For this review, take the finished solid that the model builds, in its own axes (mm). Give positions to 0.01 mm unless a question says otherwise; leave off trailing zeros. Order: outer loops, then holes, each group sorted by start corner. A loop starts at its lowest first (then second) coordinate and runs counter-clockwise, first axis right, second up. Notation, with made-up numbers: (38.25, 12.25) -> (80.25, 12.25) arc R26 cw to (80.25, 28.25) -> close; hole circle Ø10 at (-6.75, -34). An arc over 180 degrees is marked (long way). One line per item, written item: value. Start each with the question number.
from build123d import *

# Parameters (mm, degrees)
F0_R     = 38.1
F1_DEPTH = 101.6
F2_T     = -2.54


# Not quite as in the source:
# - a fillet or chamfer that OpenCascade refuses, or shapes differently, is made with other operations: its cross-section is extruded or revolved along the edge and cut away or added


with BuildPart() as f1:
    # F0 (on Top) → F1 (new body)
    with BuildSketch(Plane.XY):
        Circle(F0_R)
    extrude(amount=F1_DEPTH)

    # F2
    f2_openings = [f1.faces().sort_by_distance(p)[0] for p in [
        (0, 0, 101.6),
    ]]
    offset(amount=F2_T, openings=f2_openings)

    # F3: fillet of radius 5.08 on 1 edges, made by hand

    # F3_s1 → F3_t2 (revolve, cut)
    with BuildSketch(Plane.XZ):
        with BuildLine():
            ThreePointArc((38.1, 97.2005909488), (37.4194090512, 99.7405909488), (35.56, 101.6))
            Line((35.56, 101.6), (38.1, 101.6))
            Line((38.1, 101.6), (38.1, 97.2005909488))
        make_face()
    revolve(axis=Axis((0, 0, 101.6), (0, 0, 1)), mode=Mode.SUBTRACT)


solid = f1.part
Q1. Take a section at C-C (z = 15). State the section outline as (x, y) points.
Q2. Mouldability with a two-part tool opening along Y and no side actions: class faces 1 (the flat face through (-1, 1, 0)), 2 (the cylindrical face through (-30.235, -23.183, 47.92)), 3 (the flat face through (0, 0, 2.54)) as pulls with the +Y half, pulls with the -Y half, needs draft (parallel to the pull), parting line crosses it, or undercut.
Q3. For pin 1 Ø12 at (x, y) = (-25.5, 11.5) entering from -Z; pin 2 Ø4 at (y, z) = (23, 43) entering from +X; pin 3 Ø1.5 at (x, z) = (10, 24) entering from -Y; pin 4 Ø1.5 at (y, z) = (12, 48) entering from +X, all flat-tipped, find the tip position at first contact; note any pin that passes through.
Q4. For line 1 along Z through (x, y) = (1.5, -25.5); line 2 along X through (y, z) = (25, 8.5); line 3 along X through (y, z) = (15.5, 7.5), list the stretches that pass through material, from the lowest coordinate up.
Q5. Take a section at A-A (y = 0). State the section outline as (x, z) points.
Answers below:
1. outline: circle Ø76.2 at (0, 0); hole circle Ø71.12 at (0, 0)
2. face 1: needs draft
2. face 2: parting line crosses it
2. face 3: undercut
3. pin 1: stops at z = 0
3. pin 2: stops at x = 31.79
3. pin 3: stops at y = -36.96
3. pin 4: stops at x = 36.4
4. line 1: z = 0 to 2.54
4. line 2: x = -28.75 to -25.29, 25.29 to 28.75
4. line 3: x = -34.8 to -32, 32 to 34.8
5. outline: (-38.1, 0) -> (38.1, 0) -> (38.1, 97.2) arc R5.08 ccw to (35.56, 101.6) -> (35.56, 2.54) -> (-35.56, 2.54) -> (-35.56, 101.6) arc R5.08 ccw to (-38.1, 97.2) -> close
